```python
from build123d import *

# Parameters (mm, degrees)
EXTRUDE_1_DEPTH     = 10
EXTRUDE_2_DEPTH     = 50
SKETCH_3_R          = 10
CUT_EXTRUDE_1_DEPTH = 107.514235114
SKETCH_4_R          = 10
CUT_EXTRUDE_2_DEPTH = 101.948347169


with BuildPart() as part:
    # Sketch 1 → Extrude 1 (new body)
    with BuildSketch(Plane(origin=(0, 0, 0), x_dir=(1, 0, 0), z_dir=(0, 1, 0))):
        with BuildLine():
            Line((-28.57662693, 32.430036501), (-37.728647462, -22.372159091))
            Line((-37.728647462, -22.372159091), (12.271352538, -22.372159091))
            Line((12.271352538, -22.372159091), (24.529536474, -9.872159091))
            Line((24.529536474, -9.872159091), (12.397884427, 2.024802688))
            ThreePointArc((12.397884427, 2.024802688), (-8.714784455, 1.918154099), (-9.020536662, 23.028878313))
            Line((-9.020536662, 23.028878313), (-25.258695646, 38.952905482))
            ThreePointArc((-25.258695646, 38.952905482), (-27.419053284, 35.946509717), (-28.57662693, 32.430036501))
        make_face()
        with BuildLine():
            Line((12.397884427, 2.024802688), (24.529536474, -9.872159091))
            Line((24.529536474, -9.872159091), (36.78772041, 2.627840909))
            Line((36.78772041, 2.627840909), (36.78772041, 52.627840909))
            Line((36.78772041, 52.627840909), (-17.849431841, 42.537166231))
            ThreePointArc((-17.849431841, 42.537166231), (-21.865938759, 41.389733446), (-25.258695646, 38.952905482))
            Line((-25.258695646, 38.952905482), (-9.020536662, 23.028878313))
            ThreePointArc((-9.020536662, 23.028878313), (7.394686788, 26.540494431), (16.78772041, 12.627840909))
            ThreePointArc((16.78772041, 12.627840909), (15.646877315, 6.88991708), (12.397884427, 2.024802688))
        make_face()
    extrude(amount=EXTRUDE_1_DEPTH)

    # Sketch 1_3 → Extrude 2 (add)
    with BuildSketch(Plane(origin=(0, 0, 0), x_dir=(1, 0, 0), z_dir=(0, 1, 0))):
        with BuildLine():
            Line((-45.728647462, -20.760800889), (-37.728647462, -22.372159091))
            Line((-37.728647462, -22.372159091), (-28.57662693, 32.430036501))
            ThreePointArc((-28.57662693, 32.430036501), (-27.419053284, 35.946509717), (-25.258695646, 38.952905482))
            Line((-25.258695646, 38.952905482), (-31.290854512, 44.868370514))
            ThreePointArc((-31.290854512, 44.868370514), (-34.211631919, 40.819697763), (-35.799091446, 36.086552513))
            Line((-35.799091446, 36.086552513), (-45.728647462, -20.760800889))
        make_face()
        with BuildLine():
            Line((-31.290854512, 44.868370514), (-25.258695646, 38.952905482))
            ThreePointArc((-25.258695646, 38.952905482), (-21.865938759, 41.389733446), (-17.849431841, 42.537166231))
            Line((-17.849431841, 42.537166231), (36.78772041, 52.627840909))
            Line((36.78772041, 52.627840909), (34.234475122, 60.209459371))
            Line((34.234475122, 60.209459371), (-22.484150231, 49.56919577))
            ThreePointArc((-22.484150231, 49.56919577), (-27.248578411, 47.895236686), (-31.290854512, 44.868370514))
        make_face()
    extrude(amount=EXTRUDE_2_DEPTH)

    # Sketch 3 → Cut-Extrude 1 (cut, through all)
    with BuildSketch(Plane(origin=(-40.855844778, 0, -7.136311104), x_dir=(-0.17206538860383633, 0, 0.9850855303193783), z_dir=(-0.9850855303193784, 0, -0.17206538860383633))):
        with Locations((-1.680517951, 30)):
            Circle(SKETCH_3_R)
    extrude(amount=-CUT_EXTRUDE_1_DEPTH, mode=Mode.SUBTRACT)

    # Sketch 4 → Cut-Extrude 2 (cut, through all)
    with BuildSketch(Plane(origin=(-9.747294738, 0, -51.95859606), x_dir=(-0.9828548523659901, 0, 0.18438096208835575), z_dir=(-0.18438096208835575, 0, -0.9828548523659901))):
        with Locations((-14.748998038, 30)):
            Circle(SKETCH_4_R)
    extrude(amount=-CUT_EXTRUDE_2_DEPTH, mode=Mode.SUBTRACT)


solid = part.part
```
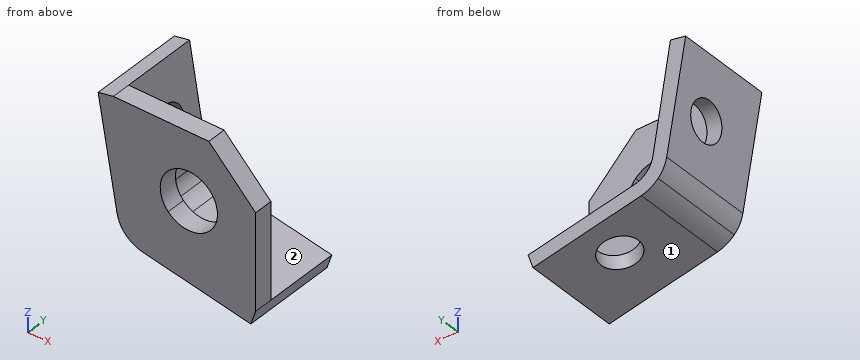
Here's how the part is built. I have some questions about the finished solid (model axes, mm). Face numbers are marked on the shaded views. A direction names the side the tool comes from. Round coordinates to 2 decimals unless told otherwise and drop trailing zeros. Write each loop counter-clockwise with the first axis right and the second up, starting at its lowest first coordinate (ties: lowest second). Pieces come first, ordered by that corner, then holes.
Q1. Will these pins go through, and if not, where does the flat tip stop? P1, Ø3, axis at y = 25, z = -1, coming from the -X side; P2, Ø3, axis at x = -25, y = 18.5, coming from the -Z side; P3, Ø3, axis at x = 6.5, z = -34, coming from the +Y side.
Q2. If we section it at B-B on y = 45: Write out the boundary of the cut face in (x, z), plus the area to 3 significant figures.
Q3. If we section it at C-C on x = 21: Write out the boundary of the cut face in (y, z), plus the area to 3 significant figures.
Q4. If we section it at A-A on y = 35: Write out the boundary of the cut face in (x, z), plus the area to 3 significant figures.
Q5. Which directions (+Z, -Z, +X, -X, +Y, -Y) give clear straight access to the entire face, cutting with the end or side of a thin tool? Please do the marked faces 1 and 2.
Q6. If we section it at D-D on z = 11.5: Write out the boundary of the cut face in (x, y), plus the area to 3 significant figures.
Q7. Please list where these lines run through material, in increasing order: probe 1 along Y at (x, z) = (-39.5, -11.5); probe 2 along Y at (x, z) = (-10.5, -30); probe 3 along Y at (x, z) = (-32, -13.5).
Answer below:
1. P1: stops at x = -42.19
1. P2: stops at z = -49.35
1. P3: stops at y = 10
2. outline: (-45.73, 20.76) - (-35.8, -36.09) arc R16.63 ccw to (-22.48, -49.57) - (34.23, -60.21) - (36.79, -52.63) - (-17.85, -42.54) arc R12.18 cw to (-28.58, -32.43) - (-37.73, 22.37) - close
2. area: 1,040 mm2
3. outline: (0, -57.73) - (50, -57.73) - (50, -49.71) - (10, -49.71) - (10, 13.47) - (0, 13.47) - close
3. area: 1,030 mm2
4. outline: (-45.73, 20.76) - (-42.06, -0.26) - (-34.18, 1.12) - (-37.73, 22.37) - close; (-39.08, -17.32) - (-35.8, -36.09) arc R16.63 ccw to (-22.48, -49.57) - (-3.76, -53.08) - (-2.32, -45.4) - (-17.85, -42.54) arc R12.18 cw to (-28.58, -32.43) - (-31.33, -15.97) - close; (13.26, -56.27) - (34.23, -60.21) - (36.79, -52.63) - (14.71, -48.55) - close
4. area: 768 mm2
5. face 1: -Z, -X, +Y, -Y
5. face 2: +Z, +X, +Y
6. outline: (-44.11, 0) - (22.93, 0) - (22.93, 10) - (-35.91, 10) - (-35.91, 50) - (-44.11, 50) - close
6. area: 998 mm2
7. probe 1: y = 0 to 20.42, 39.58 to 50
7. probe 2: y = 0 to 10
7. probe 3: y = 0 to 22.09, 37.91 to 50
